Work out the finished part from the listing and answer in its coordinate system (mm). A direction names the side the tool comes from. Round coordinates to 2 decimals unless told otherwise and drop trailing zeros. One line per item, written item: value.
Autodesk Inventor part; units mm, degrees
ref_plane "YZ Plane" through (0, 0, 0) normal (1, 0, 0) x (0, 1, 0)
ref_plane "XZ Plane" through (0, 0, 0) normal (0, 1, 0) x (-1, 0, 0)
ref_plane "XY Plane" through (0, 0, 0) normal (0, 0, 1) x (1, 0, 0)
sketch "Esboço2" plane through (0, 0, 0) normal (0, 1, 0) x (-1, 0, 0)
  line L0 (-33.3088, 0) -> (-92.4, 0)
  line L1 (-92.4, 0) -> (-92.4, -20.4)
  line L2 (-92.4, -20.4) -> (-33.3088, -20.4)
  line L3 (-38.4, -19.2) -> (-92.4, -19.2)
  line L4 (-92.4, -1.2) -> (-38.4, -1.2)
  circle A0 centre (-38.4, -10.2) radius 9
  line L5 (-47.4, -20.4) -> (-47.4, -19.2)
  line L6 (-47.4, -1.2) -> (-47.4, 0)
  arc A1 (-33.3088, -20.4) -> (-33.3088, 0) centre (-38.4, -10.2) ccw
  arc A2 (-38.4, -20.4) -> (-38.4, 0) centre (-38.4, -10.2) ccw
  line L7 (-33.3088, 0) -> (0, 0)
  line L8 (0, 0) -> (0, -20.4)
  line L9 (0, -20.4) -> (-33.3088, -20.4)
  circle A3 centre (-13.5, -10.2) radius 9
  point P0 (0, -10.2)
  point P1 (-33.3088, -20.4)
  dimension "d6" = 20.4
  dimension "d8" = 1.2
  dimension "d11" = 1.2
  dimension "d25" = 18
  dimension "d44" = 1.2
  dimension "d45" = 1.2
  dimension "d46" = 54
  dimension "d47" = 27
  dimension "d48" = 18
  dimension "d49" = 13.5
extrude "Extrusão1" add sketch "Esboço2" against normal blind 1.2 contours A1 L2 A2 L0 | L7 L8 L9 A1 | A2 L2 L5 L3 A0 L4 L6 L0 | L6 L4 L1 L0 | L4 A0 L3 L1 | L2 L1 L3 L5 | A0 | A3
extrude "Extrusão2" add sketch "Esboço2" along normal blind 9 contours L7 L8 L9 A1 | A2 L2 L5 L3 A0 L4 L6 L0 | L6 L4 L1 L0 | L2 L1 L3 L5
fillet "Arredondamento6" radius 9 4 edges at (65.4, 0, -1.2) (65.4, 0, -19.2) (29.4, 0, -10.2) (22.5, 0, -10.2)
sketch "Esboço6" plane through (0, -1.2, 0) normal (0, 0, 1) x (1, 0, 0)
  line L0 (92.4, 10.2) -> (0, 10.2)
  line L1 (0, 10.2) -> (0, 6.6)
  line L2 (0, 6.6) -> (92.4, 6.6)
  line L3 (92.4, 6.6) -> (92.4, 10.2)
  line L4 (92.4, 1.2) -> (92.4, 10.2)
  line L5 (0, 10.2) -> (0, 0)
  line L6 (38.4, 10.2) -> (92.4, 10.2)
  line L7 (38.4, 1.2) -> (92.4, 1.2)
  point P0 (0, 1.2)
  point P1 (92.4, 8.4)
  point P2 (92.4, 5.7)
  point P3 (0, 8.4)
  point P4 (0, 5.1)
  point P5 (46.2, 10.2)
  point P6 (65.4, 10.2)
  dimension "d50" = 5.4
extrude "Extrusão8" cut sketch "Esboço6" against normal up to surface (20.4 mm away)
extrude "Extrusão9" add sketch "Esboço2" along normal blind 9 contours A1 L2 A2 L0
sketch "Esboço7" plane through (0, -1.2, 0) normal (0, -1, 0) x (1, 0, 0)
  line L0 (42.3, -11.4) -> (50.1, -11.4)
  line L1 (50.1, -11.4) -> (50.1, -9)
  line L2 (50.1, -9) -> (42.3, -9)
  line L3 (42.3, -9) -> (42.3, -11.4)
  line L4 (0, 0) -> (0, -20.4)
  arc A0 (38.4, 0) -> (38.4, -20.4) centre (38.4, -10.2) ccw
  line L5 (92.4, -20.4) -> (92.4, 0)
  point P0 (42.3, -10.2)
  point P1 (0, -10.2)
  point P2 (46.2, -9)
  point P3 (28.2, -10.2)
  dimension "d56" = 7.8
  dimension "d57" = 2.4
  dimension "d76" = 42.3
  dimension "d77" = 42.3
extrude "Extrusão10" add sketch "Esboço7" along normal blind 5.4
sketch "Esboço8" plane through (42.3, -1.2, -9) normal (0, 0, 1) x (1, 0, 0)
  circle A0 centre (3.9, -2.7) radius 1.5
  line L0 (50.1, 0) -> (-42.3, 0)
  line L1 (7.8, 0) -> (7.8, -5.4)
  line L2 (0, 0) -> (0, -5.4)
  line L3 (7.8, -5.4) -> (0, -5.4)
  line L4 (7.8, -5.4) -> (0, -5.4)
  arc A1 (1.2, -2.7) -> (6.6, -2.7) centre (3.9, -2.7) ccw
  line L5 (1.2, -2.7) -> (1.2, -1.2)
  line L6 (6.6, -2.7) -> (6.6, -1.2)
  line L7 (0, 0) -> (0, 0)
  line L8 (7.8, 0) -> (7.8, 0)
  arc A2 (1.2, -1.2) -> (0, 0) centre (0, -1.2) ccw
  arc A3 (7.8, 0) -> (6.6, -1.2) centre (7.8, -1.2) ccw
  line L9 (0, 0) -> (7.8, 0)
  point P0 (-42.3, 1.2)
  point P1 (3.9, 0)
  point P2 (1.2, 0)
  point P3 (6.6, 0)
  point P4 (1.2, 0)
  point P5 (6.6, 0)
  point P6 (3.9, -5.4)
  point P7 (3.9, 0)
  dimension "d60" = 3
  dimension "d61" = 2.7
  dimension "d63" = 1.2
  dimension "d64" = 1.2
extrude "Extrusão11" cut sketch "Esboço8" against normal up to surface (2.4 mm away) contours A0 | L1 L3 A1 L6 A3 | A2 L5 A1 L3 L2
equation "\"d6\" = Diâmetro_esfera + 2 * Margem"
equation "\"d8\" = Margem"
equation "\"d11\" = Margem"
equation "\"d25\" = Diâmetro_esfera"
equation "\"d44\" = Margem"
equation "\"d45\" = Margem"
equation "\"d46\" = 3 * Diâmetro_esfera"
equation "\"d48\" = Diâmetro_esfera"
equation "\"d49\" = 0.5 * d47"
equation "\"d13\" = Margem"
equation "\"d15\" = 0.5 * Diâmetro_esfera"
equation "\"d55\" = 0.5 * Diâmetro_esfera"
equation "\"d50\" = 0.3 * Diâmetro_esfera"
equation "\"d53\" = 0.5 * Diâmetro_esfera"
equation "\"d56\" = Parafuso + 4 * Margem"
equation "\"d57\" = 2 * Margem"
equation "\"d58\" = Parafuso + 2 * Margem"
equation "\"d60\" = Parafuso"
equation "\"d61\" = 0.5 * Parafuso + Margem"
equation "\"d63\" = Margem"
equation "\"Diâmetro_esfera\" = 18"
equation "\"Margem\" = 3 * Filamento"
equation "\"Filamento\" = 0.4"
equation "\"Parafuso\" = 3"
equation "\"d42\" = Margem"
equation "\"d43\" = Margem"
equation "\"Tamanho_receptor\" = 37.257"
properties part number "Trilho 60 minutos  - 12 horas" material "Plástico PET"
(1) Flat-ended cylindrical pins translate along their axes: pin 1 Ø2 at (x, z) = (80.5, -13.5) entering from +Y; pin 2 Ø4.5 at (x, y) = (46, -4) entering from +Z; pin 3 Ø4 at (x, z) = (61.5, -7.5) entering from -Y; pin 4 Ø2.5 at (x, y) = (46.2, -3.9) entering from -Z. Find the tip coordinate at first contact, or state that the pin passes through.
Reported:
pin 1: stops at y = 1.09
pin 2: stops at z = -9
pin 3: stops at y = -1.2
pin 4: passes through
(2) A tool of negligible diameter and unlimited length cuts with its end or side. For faces 1 (the face through (48.9, -3, -10)), 2 (the face through (28.2, 7.2, -10)), 3 (the face through (43.5, -3, -10)), from which of +Z, -Z, +X, -X, +Y, -Y can it reach the whole face along a straight path? Write none if from no direction.
Reported:
face 1: +Z, -Z, +X, -Y
face 2: +X, +Y
face 3: +Z, -Z, -X, -Y
(3) Consider probe 1 along Y at (x, z) = (46.2, -10.7); probe 2 along X at (y, z) = (5, -14); probe 3 along Y at (x, z) = (51, -18.75). Determine where each line is inside the solid, lowest interval first.
Reported:
probe 1: y = -6.6 to -5.4, -2.4 to 0.01
probe 2: x = 0 to 6.39, 20.61 to 31.29
probe 3: y = -1.2 to 5.4
(4) For a pull along Z with two mould halves and no side action, classify faces 4 (the face through (60.2, 5.4, -1.8)), 5 (the face through (20, 5.4, -3)), 6 (the face through (46, 3, 0)) as pulls with the +Z half, pulls with the -Z half, needs draft (parallel to the pull), parting line crosses it, or undercut.
Reported:
face 4: undercut
face 5: needs draft
face 6: pulls with the +Z half
